```python
from build123d import *

# Parameters (mm, degrees)
F0_W        = 2.3
F0_H        = 2.3
F0_R        = 0.75
F1_DEPTH    = 10
F2_T1_DEPTH = 4.8


# Not quite as in the source:
# - a fillet or chamfer that OpenCascade refuses, or shapes differently, is made with other operations: its cross-section is extruded or revolved along the edge and cut away or added


with BuildPart() as f1:
    # F0 (on Top) → F1 (new body)
    with BuildSketch(Plane.XY):
        Rectangle(F0_W, F0_H)
        Circle(F0_R, mode=Mode.SUBTRACT)
    extrude(amount=F1_DEPTH)

    # F2: fillet of radius 0.5 on 4 edges, made by hand

    # F2_s2 → F2_t1 (cut)
    with BuildSketch(Plane.XZ.offset(-2.4)):
        with BuildLine():
            ThreePointArc((1.15, 9.5), (1.0035533906, 9.8535533906), (0.65, 10))
            Line((0.65, 10), (1.15, 10))
            Line((1.15, 10), (1.15, 9.5))
        make_face()
        with BuildLine():
            ThreePointArc((-1.15, 9.5), (-1.0035533906, 9.8535533906), (-0.65, 10))
            Line((-0.65, 10), (-1.15, 10))
            Line((-1.15, 10), (-1.15, 9.5))
        make_face()
        with BuildLine():
            ThreePointArc((1.15, 0.5), (1.0035533906, 0.1464466094), (0.65, 0))
            Line((0.65, 0), (1.15, 0))
            Line((1.15, 0), (1.15, 0.5))
        make_face()
        with BuildLine():
            ThreePointArc((-1.15, 0.5), (-1.0035533906, 0.1464466094), (-0.65, 0))
            Line((-0.65, 0), (-1.15, 0))
            Line((-1.15, 0), (-1.15, 0.5))
        make_face()
    extrude(amount=F2_T1_DEPTH, mode=Mode.SUBTRACT)


solid = f1.part
```
Can you work these out from the model? Positions are in its coordinate system, mm. Coordinates: 2 decimals unless noted, no trailing zeros. Order: outer loops, then holes, each group sorted by start corner. A loop starts at its lowest first (then second) coordinate and runs counter-clockwise, first axis right, second up. Notation, with made-up numbers: (62.5, 46.25) - (86.5, 46.25) arc R19 cw to (86.5, 74.25) - close; hole circle Ø3 at (40.25, -14.75). An arc over 180 degrees is marked (long way). Answer in a Markdown table with one row per item.
1. Suppose I cut it at C-C (z = 8.5). Please give me the cut outline in (x, y).
Reply:
| item | result |
|---|---|
| outline | (-1.15, -1.15) - (1.15, -1.15) - (1.15, 1.15) - (-1.15, 1.15) - close; hole circle Ø1.5 at (0, 0) |
2. Suppose I cut it at D-D (y = -0.55). Please give me the cut outline in (x, z), and give its area (3 significant figures).
Reply:
| item | result |
|---|---|
| outline | (-1.15, 0.5) arc R0.5 ccw to (-0.65, 0) - (-0.51, 0) - (-0.51, 10) - (-0.65, 10) arc R0.5 ccw to (-1.15, 9.5) - close; (0.51, 0) - (0.65, 0) arc R0.5 ccw to (1.15, 0.5) - (1.15, 9.5) arc R0.5 ccw to (0.65, 10) - (0.51, 10) - close |
| area | 12.6 mm^2 |
3. If I drill on line 1 along Y through (x, z) = (0, 7); line 2 along Y through (x, z) = (0.4, 7.25), over which ranges is the centre line in solid material (lowest first)?
Reply:
| item | result |
|---|---|
| line 1 | y = -1.15 to -0.75, 0.75 to 1.15 |
| line 2 | y = -1.15 to -0.63, 0.63 to 1.15 |
4. Suppose I cut it at A-A (x = 0). Please give me the cut outline in (y, z), and give its area (3 significant figures).
Reply:
| item | result |
|---|---|
| outline | (-1.15, 0) - (-0.75, 0) - (-0.75, 10) - (-1.15, 10) - close; (0.75, 0) - (1.15, 0) - (1.15, 10) - (0.75, 10) - close |
| area | 8.00 mm^2 |
5. If we mould it in two halves opening along Y, with no side actions, what happens to faces 1 (the flat face through (0, 1.15, 5)), 2 (the cylindrical face through (-0.75, 0.03, 4.93)), 3 (the flat face through (0, -1.15, 5))? For each: pulls with the +Y half, pulls with the -Y half, needs draft (parallel to the pull), parting line crosses it, or undercut.
Reply:
| item | result |
|---|---|
| face 1 | pulls with the +Y half |
| face 2 | undercut |
| face 3 | pulls with the -Y half |
6. Suppose I cut it at B-B (y = 0.1). Please give me the cut outline in (x, z).
Reply:
| item | result |
|---|---|
| outline | (-1.15, 0.5) arc R0.5 ccw to (-0.74, 0.01) - (-0.74, 9.99) arc R0.5 ccw to (-1.15, 9.5) - close; (0.74, 0.01) arc R0.5 ccw to (1.15, 0.5) - (1.15, 9.5) arc R0.5 ccw to (0.74, 9.99) - close |
